```python
from build123d import *

# Parameters (mm, degrees)
BOSS_EXTRUDE1_DEPTH = 6.35


with BuildPart() as part:
    # Sketch1 → Boss-Extrude1 (new body)
    with BuildSketch(Plane.XY):
        with BuildLine():
            Line((63.5, 6.35), (63.5, 19.05))
            Line((63.5, 19.05), (69.85, 19.05))
            Line((69.85, 19.05), (69.85, 57.15))
            Line((69.85, 57.15), (63.5, 57.15))
            Line((63.5, 57.15), (63.5, 82.55))
            ThreePointArc((63.5, 82.55), (0, 44.45), (-63.5, 82.55))
            Line((-63.5, 82.55), (-63.5, 57.15))
            Line((-63.5, 57.15), (-69.85, 57.15))
            Line((-69.85, 57.15), (-69.85, 19.05))
            Line((-69.85, 19.05), (-63.5, 19.05))
            Line((-63.5, 19.05), (-63.5, 6.35))
            Line((-63.5, 6.35), (-38.1, 6.35))
            Line((-38.1, 6.35), (-38.1, 0))
            Line((-38.1, 0), (-12.7, 0))
            Line((-12.7, 0), (-12.7, 6.35))
            Line((-12.7, 6.35), (12.7, 6.35))
            Line((12.7, 6.35), (12.7, 0))
            Line((12.7, 0), (38.1, 0))
            Line((38.1, 0), (38.1, 6.35))
            Line((38.1, 6.35), (63.5, 6.35))
        make_face()
    extrude(amount=BOSS_EXTRUDE1_DEPTH)


solid = part.part
```
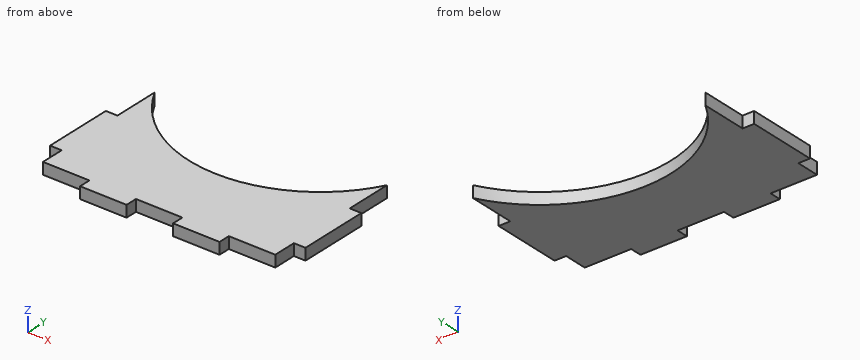
Source: CAD feature listing. Evaluate the final solid. Frame: model axes, mm. Give positions to 0.01 mm unless a question says otherwise; leave off trailing zeros. Order: outer loops, then holes, each group sorted by start corner. A loop starts at its lowest first (then second) coordinate and runs counter-clockwise, first axis right, second up. Notation, with made-up numbers: (-6, -1.75) -> (2, -1.75) arc R19 ccw to (2, 15.25) -> close; hole circle Ø10 at (-10, 17.5). An arc over 180 degrees is marked (long way). Use a Markdown table: item, result.
Q1. Section A-A (y = 70). Return the cut outline in (x, z), and give its area (3 significant figures).
A:
| item | result |
|---|---|
| outline | (-63.5, 0) -> (-55, 0) -> (-55, 6.35) -> (-63.5, 6.35) -> close; (55, 0) -> (63.5, 0) -> (63.5, 6.35) -> (55, 6.35) -> close |
| area | 108 mm^2 |
Q2. Section D-D (x = 1). Return the cut outline in (y, z), and give its area (3 significant figures).
A:
| item | result |
|---|---|
| outline | (6.35, 0) -> (44.46, 0) -> (44.46, 6.35) -> (6.35, 6.35) -> close |
| area | 242 mm^2 |
Q3. First-contact query: P1, Ø3, axis at x = 50, z = 4, coming from the -Y side; P2, Ø3, axis at x = -67, z = 3, coming from the +Y side; P3, Ø3, axis at y = 10.5, z = 3.5, coming from the -X side. Flat tips, straight axial feed; report the tip coordinate or a pass-through.
A:
| item | result |
|---|---|
| P1 | y = 6.35 |
| P2 | y = 57.15 |
| P3 | x = -63.5 |
Q4. Section C-C (y = 11). Return the cut outline in (x, z), and give its area (3 significant figures).
A:
| item | result |
|---|---|
| outline | (-63.5, 0) -> (63.5, 0) -> (63.5, 6.35) -> (-63.5, 6.35) -> close |
| area | 806 mm^2 |
Q5. Section B-B (z = 4.75). Return the cut outline in (x, y), and give its area (3 significant figures).
A:
| item | result |
|---|---|
| outline | (-69.85, 19.05) -> (-63.5, 19.05) -> (-63.5, 6.35) -> (-38.1, 6.35) -> (-38.1, 0) -> (-12.7, 0) -> (-12.7, 6.35) -> (12.7, 6.35) -> (12.7, 0) -> (38.1, 0) -> (38.1, 6.35) -> (63.5, 6.35) -> (63.5, 19.05) -> (69.85, 19.05) -> (69.85, 57.15) -> (63.5, 57.15) -> (63.5, 82.55) arc R71.97 cw to (-63.5, 82.55) -> (-63.5, 57.15) -> (-69.85, 57.15) -> close |
| area | 7,040 mm^2 |
Q6. Material intervals for line 1 (X direction, y = 6, z = 4.75); line 2 (X direction, y = 18.5, z = 5.25); line 3 (X direction, y = 61, z = 2.5), sorted ascending. Write a range as [from, to].
A:
| item | result |
|---|---|
| line 1 | [-38.1, -12.7], [12.7, 38.1] |
| line 2 | [-63.5, 63.5] |
| line 3 | [-63.5, -45.92], [45.92, 63.5] |
